Part model, mm, in its own coordinate system. Round coordinates to 2 decimals unless told otherwise and drop trailing zeros. Loops run counter-clockwise (first coordinate to the right, second up) from the corner with the lowest first, then second, coordinate; pieces in that order, holes last.
(1) Probe probe 1 along Z at (x, y) = (-32, 3.7); probe 2 along X at (y, z) = (1.55, 18); probe 3 along X at (y, z) = (4.5, 0). List the from-to ranges inside material, lowest first.
(2) Cut at A-A on z = 0. List the corners of the cut face in (x, y).
(3) Cut at C-C on x = 32. List the corners of the cut face in (y, z).
(4) Cut at D-D on y = 1.8. Count the separate pieces of the cut face and the enclosed holes in it, then the cut area to 3 significant figures.
(5) Flat gauge pins, fed straight in: pin 1 (2.5 mm diameter, centred on x = 25, z = -18, fed in from +Y); pin 2 (3 mm diameter, centred on y = 3, z = -39, fed in from -X); pin 3 (1.5 mm diameter, centred on y = 2, z = -2, fed in from +X); pin 4 (6.5 mm diameter, centred on x = -32, z = 43.74, fed in from -Y). Where does each tip first touch, or does it go through?
(6) Cut at B-B on x = 0. List the corners of the cut face in (y, z), then the cut area to 3 significant figures.
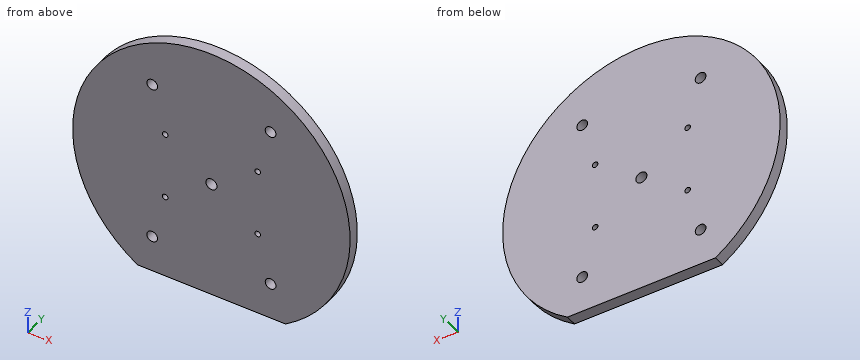
from build123d import *

# Parameters (mm, degrees)
SKETCH1_R           = 75
BOSS_EXTRUDE1_DEPTH = 6
SKETCH2_R           = 2.9
SKETCH2_R_2         = 3
SKETCH2_R_3         = 1.5
SKETCH2_W           = 80
SKETCH2_H           = 23.30375559
CUT_EXTRUDE1_DEPTH  = 6


with BuildPart() as part:
    # Sketch1 → Boss-Extrude1 (new body)
    with BuildSketch(Plane(origin=(0, 0, 0), x_dir=(1, 0, 0), z_dir=(0, 1, 0))):
        Circle(SKETCH1_R)
    extrude(amount=BOSS_EXTRUDE1_DEPTH)

    # Sketch2 → Cut-Extrude1 (cut)
    with BuildSketch(Plane(origin=(0, 6, 0), x_dir=(1, 0, 0), z_dir=(0, 1, 0))):
        with Locations((-32, 43.742887702)):
            Circle(SKETCH2_R)
        with Locations((32, 43.742887702)):
            Circle(SKETCH2_R)
        Circle(SKETCH2_R_2)
        with Locations((-32, -43.742887702)):
            Circle(SKETCH2_R)
        with Locations((32, -43.742887702)):
            Circle(SKETCH2_R)
        with Locations((25, 18)):
            Circle(SKETCH2_R_3)
        with Locations((-25, 18)):
            Circle(SKETCH2_R_3)
        with Locations((-25, -18)):
            Circle(SKETCH2_R_3)
        with Locations((25, -18)):
            Circle(SKETCH2_R_3)
        with Locations((0, 75.094765497)):
            Rectangle(SKETCH2_W, SKETCH2_H)
    extrude(amount=-CUT_EXTRUDE1_DEPTH, mode=Mode.SUBTRACT)


solid = part.part
Final values:
1. probe 1: z = -63.44 to -46.64, -40.84 to 40.84, 46.64 to 67.83
1. probe 2: x = -72.81 to -26.5, -23.5 to 23.5, 26.5 to 72.81
1. probe 3: x = -75 to -3, 3 to 75
2. outline: (-75, 0) - (-3, 0) - (-3, 6) - (-75, 6) - close; (3, 0) - (75, 0) - (75, 6) - (3, 6) - close
3. outline: (0, -63.44) - (6, -63.44) - (6, -46.64) - (0, -46.64) - close; (0, -40.84) - (6, -40.84) - (6, 40.84) - (0, 40.84) - close; (0, 46.64) - (6, 46.64) - (6, 67.83) - (0, 67.83) - close
4. separate pieces: 1
4. enclosed holes: 9
4. area: 16,900 mm2
5. pin 1: passes through
5. pin 2: stops at x = -64.95
5. pin 3: stops at x = 74.99
5. pin 4: stops at y = 0
6. outline: (0, -63.44) - (6, -63.44) - (6, -3) - (0, -3) - close; (0, 3) - (6, 3) - (6, 75) - (0, 75) - close
6. area: 795 mm2
